Verification items for the finished model (mm, model axes). Face numbers are marked on the shaded views. A direction names the side the tool comes from. Give positions to 0.01 mm unless a question says otherwise; leave off trailing zeros. Order: outer loops, then holes, each group sorted by start corner. A loop starts at its lowest first (then second) coordinate and runs counter-clockwise, first axis right, second up. Notation, with made-up numbers: M 43,59 L 75,59 A22 ccw 75,78 Z; hole C 59.5,-12.5 d3. An arc over 180 degrees is marked long. Answer as a JSON object with one key per item and string values.
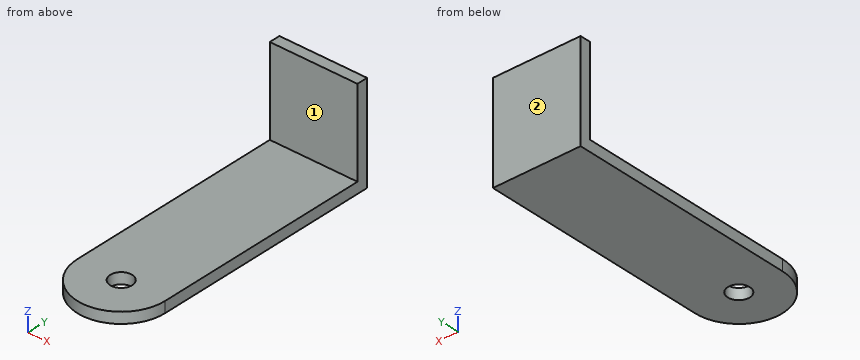
Autodesk Inventor part; units mm, degrees
ref_plane "YZ Plane" through (0, 0, 0) normal (1, 0, 0) x (0, 1, 0)
ref_plane "XZ Plane" through (0, 0, 0) normal (0, 1, 0) x (-1, 0, 0)
ref_plane "XY Plane" through (0, 0, 0) normal (0, 0, 1) x (1, 0, 0)
sketch "Sketch1" plane through (0, 0, 0) normal (0, 0, 1) x (1, 0, 0)
  circle A0 centre (0, 0) radius 12.7
  line L0 (12.7, 0) -> (12.7, 66.675)
  line L1 (-12.7, 0) -> (-12.7, 66.675)
  line L2 (-12.7, 66.675) -> (12.7, 66.675)
  circle A1 centre (0, 0) radius 3.175
  dimension "d0" = 25.4
  dimension "d1" = 66.675
  dimension "d3" = 6.35
extrude "Extrusion1" add sketch "Sketch1" along normal blind 3.175
sketch "Sketch2" plane through (0, 0, 3.175) normal (0, 0, 1) x (1, 0, 0)
  line L0 (12.7, 66.675) -> (-12.7, 66.675)
  line L1 (-12.7, 66.675) -> (12.7, 66.675)
  line L2 (12.7, 66.675) -> (12.7, 63.5)
  line L3 (12.7, 63.5) -> (-12.7, 63.5)
  line L4 (-12.7, 63.5) -> (-12.7, 66.675)
  point P0 (0, 0)
  dimension "d6" = 25.4
  dimension "d7" = 3.175
extrude "Extrusion2" add sketch "Sketch2" along normal blind 25.4
properties part number "Roller holder_CPY"
Q1. Section check D-D on x = 7.5. Record the cut outline in (y, z) (3 decimals), then the cut area to 3 significant figures.
Resolved:
{"outline": "M -10.249,0 L 66.675,0 L 66.675,28.575 L 63.5,28.575 L 63.5,3.175 L -10.249,3.175 Z", "area": "325 mm²"}
Q2. Gauge pin test, flat ends, axial feed: pin 1 Ø4 at (x, y) = (-0.5, 43) entering from +Z (3 decimals); pin 2 Ø7.5 at (x, z) = (3, 18.5) entering from -Y; pin 3 Ø12 at (y, z) = (21.5, 12.5) entering from +X. Record the tip position at first contact, or that the pin passes through.
Resolved:
{"pin 1": "stops at z = 3.175", "pin 2": "stops at y = 63.5", "pin 3": "passes through"}
Q3. Section check C-C on z = 26.75. Record the cut outline in (x, y) (3 decimals), then the cut area to 3 significant figures.
Resolved:
{"outline": "M -12.7,63.5 L 12.7,63.5 L 12.7,66.675 L -12.7,66.675 Z", "area": "80.6 mm²"}
Q4. Section check B-B on y = 34.5. Record the cut outline in (x, z) (3 decimals), then the cut area to 3 significant figures.
Resolved:
{"outline": "M -12.7,0 L 12.7,0 L 12.7,3.175 L -12.7,3.175 Z", "area": "80.6 mm²"}
Q5. Material ranges on L1, parallel to Y at x = 0, z = 2.1 (3 decimals); L2, parallel to Z at x = 2, y = 12 (3 decimals); L3, parallel to Y at x = -3.5, z = 12.75 (3 decimals), recorded low to high.
Resolved:
{"L1": "y = -12.7 to -3.175, 3.175 to 66.675", "L2": "z = 0 to 3.175", "L3": "y = 63.5 to 66.675"}
Q6. Section check A-A on x = 0. Record the cut outline in (y, z) (3 decimals).
Resolved:
{"outline": "M -12.7,0 L -3.175,0 L -3.175,3.175 L -12.7,3.175 Z; M 3.175,0 L 66.675,0 L 66.675,28.575 L 63.5,28.575 L 63.5,3.175 L 3.175,3.175 Z"}
Q7. Tool access check on the marked faces 1 and 2. Record the directions out of +Z, -Z, +X, -X, +Y, -Y that give a thin tool (end or side, any length) a straight path to the whole face; none if there is none.
Resolved:
{"face 1": "+Z, +X, -X, -Y", "face 2": "+Z, -Z, +X, -X, +Y"}
